Geometry check sheet. Reference: the model listing, model coordinates, mm. A direction names the side the tool comes from. Coordinates: 2 decimals unless noted, no trailing zeros. Write each loop counter-clockwise with the first axis right and the second up, starting at its lowest first coordinate (ties: lowest second). Pieces come first, ordered by that corner, then holes. Notation, with made-up numbers: (1, -24) -> (12, -24) arc R32 ccw to (12, 7) -> close; hole circle Ø8 at (-7.5, -26). An arc over 180 degrees is marked (long way). One line per question, with ' | ' between items.
from build123d import *

# Parameters (mm, degrees)
SKETCH1_W                       = 38.1
SKETCH1_H                       = 38.1
BOSS_EXTRUDE1_DEPTH             = 6.35
BOSS_EXTRUDE2_DEPTH             = 167.118447297
SKETCH3_W                       = 38.1
SKETCH3_H                       = 38.1
BOSS_EXTRUDE3_DEPTH             = 6.35
FILLET1_R                       = 3.175
F_1_4_0_25_DIAMETER_HOLE1_D     = 6.35
F_1_4_0_25_DIAMETER_HOLE1_DEPTH = 6.35
F_1_4_0_25_DIAMETER_HOLE2_D     = 6.35
CUT_EXTRUDE1_REACH              = 215.764


with BuildPart() as part:
    # Sketch1 → Boss-Extrude1 (new body)
    with BuildSketch(Plane(origin=(-17.28438521, -5.761461737, 3.840974491), x_dir=(-0.1956984219160322, -0.06523280730534455, -0.9784921095801634), z_dir=(0.9282791216329135, 0.3094263738776401, -0.20628424925175834))):
        Rectangle(SKETCH1_W, SKETCH1_H)
    extrude(amount=-BOSS_EXTRUDE1_DEPTH)

    # Sketch2 → Boss-Extrude2 (add)
    with BuildSketch(Plane(origin=(-23.178957633, -7.726319211, 5.150879474), x_dir=(0.19569842191603226, 0.06523280730534461, 0.9784921095801634), z_dir=(-0.9282791216329135, -0.3094263738776404, 0.20628424925175842))):
        Polygon((-19.05, 19.05), (0, 19.05), (0, 15.875), (-15.875, 15.875), (-15.875, -15.875), (0, -15.875), (0, -19.05), (-19.05, -19.05), align=None)
    extrude(amount=BOSS_EXTRUDE2_DEPTH)

    # Sketch3 → Boss-Extrude3 (add)
    with BuildSketch(Plane(origin=(-178.311523099, -59.437174366, 39.624782911), x_dir=(-0.19569842191603198, -0.0652328073053445, -0.9784921095801634), z_dir=(0.9282791216329136, 0.30942637387764027, -0.20628424925175817))):
        Rectangle(SKETCH3_W, SKETCH3_H)
    extrude(amount=BOSS_EXTRUDE3_DEPTH)

    # Fillet1
    fillet1_edges = [part.edges().sort_by_distance(p)[0] for p in [
        (-29.752429642, 6.816242738, -2.615901646),
        (-19.712198071, -23.304451975, -2.615901646),
        (-178.990422686, -42.929754944, 30.548096808),
        (-168.950191115, -73.050449657, 30.548096808),
    ]]
    fillet(fillet1_edges, radius=FILLET1_R)

    # 1/4 (0.25) Diameter Hole1
    with Locations(Plane(origin=(-17.28438521, -5.761461737, 3.840974491), x_dir=(-0.19569842191603223, -0.0652328073053446, -0.9784921095801634), z_dir=(0.9282791216329135, 0.3094263738776401, -0.20628424925175837))):
        with Locations((-12.7, 12.7), (-12.7, -12.7), (9.525, 6.35), (9.525, -6.35)):
            Hole(F_1_4_0_25_DIAMETER_HOLE1_D / 2, depth=F_1_4_0_25_DIAMETER_HOLE1_DEPTH)

    # 1/4 (0.25) Diameter Hole2 (through all)
    with Locations(Plane(origin=(-178.311523099, -59.437174366, 39.624782911), x_dir=(0.19569842191603223, 0.06523280730534461, 0.9784921095801634), z_dir=(-0.9282791216329135, -0.3094263738776401, 0.2062842492517584))):
        with Locations((12.7, 12.7), (12.7, -12.7), (-9.525, -6.35), (-9.525, 6.35)):
            Hole(F_1_4_0_25_DIAMETER_HOLE2_D / 2)

    # Sketch10 → Cut-Extrude1 (cut, up to next)
    with BuildSketch(Plane(origin=(-3.106712448, -1.035570816, -15.53356224), x_dir=(0.9806641258145292, -0.013017665386918594, -0.19526498080377744), z_dir=(0.1956984219160322, 0.06523280730534471, 0.9784921095801634)), mode=Mode.PRIVATE) as cut_extrude1_sk1:
        with BuildLine():
            Line((-26.787357564, -18.493233536), (-33.230145008, 0.419416497))
            ThreePointArc((-33.230145008, 0.419416497), (-34.032250279, 1.332050316), (-35.244753917, 1.410205802))
            Line((-35.244753917, 1.410205802), (-54.15740395, -5.032581643))
            ThreePointArc((-54.15740395, -5.032581643), (-55.229706496, -6.433165686), (-54.346087984, -7.95982437))
            Line((-54.346087984, -7.95982437), (-28.990650506, -20.429686959))
            ThreePointArc((-28.990650506, -20.429686959), (-27.24205563, -20.197556886), (-26.787357564, -18.493233536))
        make_face()
    cut_extrude1_tool1 = extrude(cut_extrude1_sk1.sketch, amount=-CUT_EXTRUDE1_REACH, mode=Mode.PRIVATE) & part.part
    # Sketch10 → Cut-Extrude1 (cut, up to next)
    with BuildSketch(Plane(origin=(-3.106712448, -1.035570816, -15.53356224), x_dir=(0.9806641258145292, -0.013017665386918594, -0.19526498080377744), z_dir=(0.1956984219160322, 0.06523280730534471, 0.9784921095801634)), mode=Mode.PRIVATE) as cut_extrude1_sk2:
        with BuildLine():
            Line((-35.001446932, -22.477326167), (-60.35688441, -10.007463578))
            ThreePointArc((-60.35688441, -10.007463578), (-62.105479286, -10.239593651), (-62.560177352, -11.943917001))
            Line((-62.560177352, -11.943917001), (-56.117389908, -30.856567035))
            ThreePointArc((-56.117389908, -30.856567035), (-55.315284637, -31.769200853), (-54.102780999, -31.847356339))
            Line((-54.102780999, -31.847356339), (-35.190130966, -25.404568895))
            ThreePointArc((-35.190130966, -25.404568895), (-34.11782842, -24.003984851), (-35.001446932, -22.477326167))
        make_face()
    cut_extrude1_tool2 = extrude(cut_extrude1_sk2.sketch, amount=-CUT_EXTRUDE1_REACH, mode=Mode.PRIVATE) & part.part
    # Sketch10 → Cut-Extrude1 (cut, up to next)
    with BuildSketch(Plane(origin=(-3.106712448, -1.035570816, -15.53356224), x_dir=(0.9806641258145292, -0.013017665386918594, -0.19526498080377744), z_dir=(0.1956984219160322, 0.06523280730534471, 0.9784921095801634)), mode=Mode.PRIVATE) as cut_extrude1_sk3:
        with BuildLine():
            Line((-62.852136119, -30.779068786), (-69.294923563, -11.866418753))
            ThreePointArc((-69.294923563, -11.866418753), (-70.097028834, -10.953784934), (-71.309532471, -10.875629448))
            Line((-71.309532471, -10.875629448), (-90.222182505, -17.318416892))
            ThreePointArc((-90.222182505, -17.318416892), (-91.294485051, -18.719000936), (-90.410866539, -20.24565962))
            Line((-90.410866539, -20.24565962), (-65.055429061, -32.715522209))
            ThreePointArc((-65.055429061, -32.715522209), (-63.306834185, -32.483392136), (-62.852136119, -30.779068786))
        make_face()
    cut_extrude1_tool3 = extrude(cut_extrude1_sk3.sketch, amount=-CUT_EXTRUDE1_REACH, mode=Mode.PRIVATE) & part.part
    # Sketch10 → Cut-Extrude1 (cut, up to next)
    with BuildSketch(Plane(origin=(-3.106712448, -1.035570816, -15.53356224), x_dir=(0.9806641258145292, -0.013017665386918594, -0.19526498080377744), z_dir=(0.1956984219160322, 0.06523280730534471, 0.9784921095801634)), mode=Mode.PRIVATE) as cut_extrude1_sk4:
        with BuildLine():
            Line((-71.066225487, -34.763161417), (-96.421662965, -22.293298828))
            ThreePointArc((-96.421662965, -22.293298828), (-98.170257841, -22.525428901), (-98.624955907, -24.229752251))
            Line((-98.624955907, -24.229752251), (-92.182168463, -43.142402284))
            ThreePointArc((-92.182168463, -43.142402284), (-91.380063192, -44.055036103), (-90.167559554, -44.133191589))
            Line((-90.167559554, -44.133191589), (-71.254909521, -37.690404145))
            ThreePointArc((-71.254909521, -37.690404145), (-70.182606975, -36.289820101), (-71.066225487, -34.763161417))
        make_face()
    cut_extrude1_tool4 = extrude(cut_extrude1_sk4.sketch, amount=-CUT_EXTRUDE1_REACH, mode=Mode.PRIVATE) & part.part
    # Sketch10 → Cut-Extrude1 (cut, up to next)
    with BuildSketch(Plane(origin=(-3.106712448, -1.035570816, -15.53356224), x_dir=(0.9806641258145292, -0.013017665386918594, -0.19526498080377744), z_dir=(0.1956984219160322, 0.06523280730534471, 0.9784921095801634)), mode=Mode.PRIVATE) as cut_extrude1_sk5:
        with BuildLine():
            Line((-98.916914674, -43.064904036), (-105.359702118, -24.152254002))
            ThreePointArc((-105.359702118, -24.152254002), (-106.161807388, -23.239620184), (-107.374311026, -23.161464698))
            Line((-107.374311026, -23.161464698), (-126.28696106, -29.604252142))
            ThreePointArc((-126.28696106, -29.604252142), (-127.359263606, -31.004836186), (-126.475645094, -32.531494869))
            Line((-126.475645094, -32.531494869), (-101.120207616, -45.001357459))
            ThreePointArc((-101.120207616, -45.001357459), (-99.371612739, -44.769227386), (-98.916914674, -43.064904036))
        make_face()
    cut_extrude1_tool5 = extrude(cut_extrude1_sk5.sketch, amount=-CUT_EXTRUDE1_REACH, mode=Mode.PRIVATE) & part.part
    # Sketch10 → Cut-Extrude1 (cut, up to next)
    with BuildSketch(Plane(origin=(-3.106712448, -1.035570816, -15.53356224), x_dir=(0.9806641258145292, -0.013017665386918594, -0.19526498080377744), z_dir=(0.1956984219160322, 0.06523280730534471, 0.9784921095801634)), mode=Mode.PRIVATE) as cut_extrude1_sk6:
        with BuildLine():
            Line((-107.131004042, -47.048996667), (-132.48644152, -34.579134078))
            ThreePointArc((-132.48644152, -34.579134078), (-134.235036396, -34.811264151), (-134.689734462, -36.5155875))
            Line((-134.689734462, -36.5155875), (-128.246947018, -55.428237534))
            ThreePointArc((-128.246947018, -55.428237534), (-127.444841747, -56.340871353), (-126.232338109, -56.419026839))
            Line((-126.232338109, -56.419026839), (-107.319688075, -49.976239394))
            ThreePointArc((-107.319688075, -49.976239394), (-106.247385529, -48.575655351), (-107.131004042, -47.048996667))
        make_face()
    cut_extrude1_tool6 = extrude(cut_extrude1_sk6.sketch, amount=-CUT_EXTRUDE1_REACH, mode=Mode.PRIVATE) & part.part
    # Sketch10 → Cut-Extrude1 (cut, up to next)
    with BuildSketch(Plane(origin=(-3.106712448, -1.035570816, -15.53356224), x_dir=(0.9806641258145292, -0.013017665386918594, -0.19526498080377744), z_dir=(0.1956984219160322, 0.06523280730534471, 0.9784921095801634)), mode=Mode.PRIVATE) as cut_extrude1_sk7:
        with BuildLine():
            Line((-134.981693228, -55.350739286), (-141.424480673, -36.438089252))
            ThreePointArc((-141.424480673, -36.438089252), (-142.226585943, -35.525455434), (-143.439089581, -35.447299948))
            Line((-143.439089581, -35.447299948), (-162.351739615, -41.890087392))
            ThreePointArc((-162.351739615, -41.890087392), (-163.424042161, -43.290671435), (-162.540423649, -44.817330119))
            Line((-162.540423649, -44.817330119), (-137.184986171, -57.287192709))
            ThreePointArc((-137.184986171, -57.287192709), (-135.436391294, -57.055062636), (-134.981693228, -55.350739286))
        make_face()
    cut_extrude1_tool7 = extrude(cut_extrude1_sk7.sketch, amount=-CUT_EXTRUDE1_REACH, mode=Mode.PRIVATE) & part.part
    # Sketch10 → Cut-Extrude1 (cut, up to next)
    with BuildSketch(Plane(origin=(-3.106712448, -1.035570816, -15.53356224), x_dir=(0.9806641258145292, -0.013017665386918594, -0.19526498080377744), z_dir=(0.1956984219160322, 0.06523280730534471, 0.9784921095801634)), mode=Mode.PRIVATE) as cut_extrude1_sk8:
        with BuildLine():
            Line((-143.195782597, -59.334831917), (-168.551220075, -46.864969328))
            ThreePointArc((-168.551220075, -46.864969328), (-170.299814951, -47.0970994), (-170.754513017, -48.80142275))
            Line((-170.754513017, -48.80142275), (-164.311725573, -67.714072784))
            ThreePointArc((-164.311725573, -67.714072784), (-163.509620302, -68.626706603), (-162.297116664, -68.704862089))
            Line((-162.297116664, -68.704862089), (-143.38446663, -62.262074644))
            ThreePointArc((-143.38446663, -62.262074644), (-142.312164084, -60.861490601), (-143.195782597, -59.334831917))
        make_face()
    cut_extrude1_tool8 = extrude(cut_extrude1_sk8.sketch, amount=-CUT_EXTRUDE1_REACH, mode=Mode.PRIVATE) & part.part
    add(cut_extrude1_tool1.solids().sort_by_distance((-41.341778, -9.255249, -7.338571))[0], mode=Mode.SUBTRACT)
    add(cut_extrude1_tool2.solids().sort_by_distance((-52.491569, -22.022534, -4.25746))[0], mode=Mode.SUBTRACT)
    add(cut_extrude1_tool3.solids().sort_by_distance((-76.709213, -21.044393, 0.520859))[0], mode=Mode.SUBTRACT)
    add(cut_extrude1_tool4.solids().sort_by_distance((-87.859003, -33.811679, 3.60197))[0], mode=Mode.SUBTRACT)
    add(cut_extrude1_tool5.solids().sort_by_distance((-112.076647, -32.833538, 8.380289))[0], mode=Mode.SUBTRACT)
    add(cut_extrude1_tool6.solids().sort_by_distance((-123.226438, -45.600823, 11.4614))[0], mode=Mode.SUBTRACT)
    add(cut_extrude1_tool7.solids().sort_by_distance((-147.444082, -44.622683, 16.239719))[0], mode=Mode.SUBTRACT)
    add(cut_extrude1_tool8.solids().sort_by_distance((-158.593872, -57.389968, 19.32083))[0], mode=Mode.SUBTRACT)


solid = part.part
1. Mould release check, pull along Y, two halves, no side actions. Record for faces 1 (the face through (-16.378, -5.74, 23.127)), 2 (the face through (-21.205, -10.444, -5.219)), 3 (the face through (-150.55, -50.04, 15.62)), 4 (the face through (-100.31, -33.72, 2.84)): released by +Y, released by -Y, zero draft, split by the parting line, or undercut.
Worked answers:
face 1: released by +Y | face 2: undercut | face 3: undercut | face 4: released by -Y
2. Cross-section at B-B on z = 51. Give the number of separate pieces and of enclosed holes in the cut face, and give its area (3 significant figures).
Worked answers:
separate pieces: 3 | enclosed holes: 0 | area: 166 mm²
3. Go/stop test with flat-tipped pins: P1, Ø2, axis at x = -33.5, y = -14.5, coming from the -Z side; P2, Ø5, axis at x = -130, z = 32, coming from the +Y side; P3, Ø3, axis at x = -127, z = 17, coming from the +Y side; P4, Ø1.5, axis at x = -98, z = 10.5, coming from the -Y side. Record where each tip stops, or that it passes through.
Worked answers:
P1: through | P2: y = -59.7 | P3: y = -21.75 | P4: y = -53
4. Cross-section at A-A on x = -76. Record the boundary of the cut face in (y, z).
Worked answers:
outline: (-45.41, -1.24) -> (-38.72, -1.69) -> (-38.72, 1.56) -> (-42.07, 1.78) -> (-42.07, 18) -> (-45.41, 18.23) -> close; (-33.68, -2.02) -> (-28.69, -2.36) -> (-28.16, 0.85) -> (-33.15, 1.19) -> close; (-11.95, -3.47) -> (-5.25, -3.92) -> (-5.25, 15.55) -> (-8.6, 15.77) -> (-8.6, -0.45) -> (-11.95, -0.23) -> close
5. Tool access check on faces 5 (the face through (-95.334, -51.859, 9.817)), 6 (the face through (-17.317, -5.491, 4.102)), 7 (the face through (-61.649, -21.585, -4.055)), 8 (the face through (-117.855, -25.898, 7.474)), 9 (the face through (-85.364, -28.602, 1.156)). Record the directions out of +Z, -Z, +X, -X, +Y, -Y that give a thin tool (end or side, any length) a straight path to the whole face; none if there is none.
Worked answers:
face 5: +Z, -Z, +X, -Y | face 6: -Z, +X, +Y | face 7: -Z | face 8: +Z, -Z | face 9: +Z
6. Material ranges on line 1 (Y direction, x = -82, z = 1.5); line 2 (Y direction, x = -147.5, z = 20); line 3 (Y direction, x = -76, z = 12.5), recorded low to high. Write a range as from..to.
Worked answers:
line 1: -47.41..-40.72, -30.18..-25.13, -10.6..-7.25 | line 2: -69.25..-65.9, -32.43..-29.09 | line 3: -45.41..-42.07, -8.6..-5.25
